Can you work these out from the drawing? Everything is in mm from the part's minimum corner. Give positions to 0.01 mm unless a question says otherwise; leave off trailing zeros. Loops run counter-clockwise (first coordinate to the right, second up) from the corner with the lowest first, then second, coordinate; pieces in that order, holes last.
Q1. If we section it at C-C (z = 94): Please give me the cut outline in (x, y).
Q2. I need wall thicknesses on line 1 (Y direction, x = 18, z = 3); line 2 (X direction, y = 17.5, z = 67); line 3 (X direction, y = 21, z = 73). Which ranges of each line are inside material? Lowest first, please.
Q3. If we section it at A-A (y = 18): Please give me the cut outline in (x, z).
Q4. If we section it at D-D (y = 32): Please give me the cut outline in (x, z).
Q5. If we section it at B-B (x = 20.5): Please give me the cut outline in (y, z), plus the area to 3 significant figures.
Q6. Will these pins go through, and if not, where does the flat tip stop? P1, Ø10, axis at x = 25.5, z = 93.5, coming from the +Y side; P2, Ø8, axis at x = 15.5, y = 25, coming from the -Z side; P3, Ø6, axis at y = 27.5, z = 32, coming from the -X side; P4, Ø1.5, axis at x = 32, y = 17.5, coming from the -Z side.
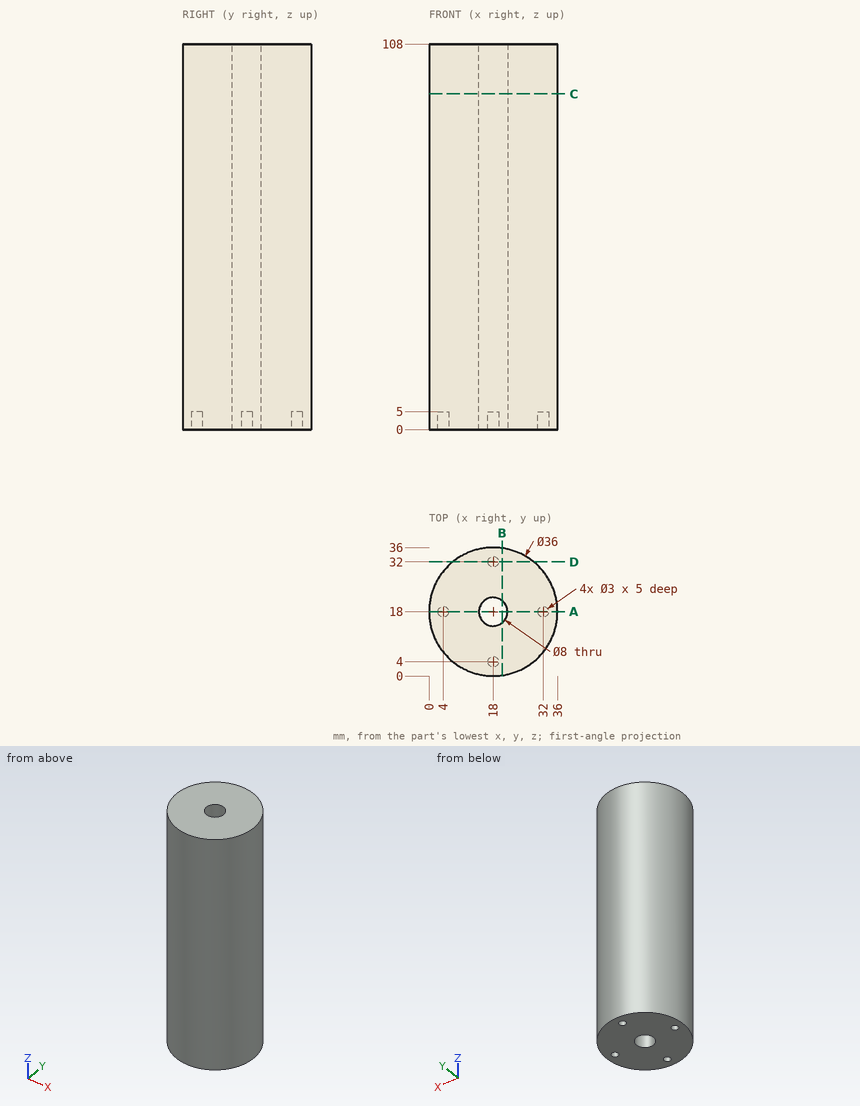
Check sheet entries:
1. outline: circle Ø36 at (18, 18); hole circle Ø8 at (18, 18)
2. line 1: y = 0 to 2.5, 5.5 to 14, 22 to 30.5, 33.5 to 36
2. line 2: x = 0.01 to 14.03, 21.97 to 35.99
2. line 3: x = 0.25 to 15.35, 20.65 to 35.75
3. outline: (0, 0) - (2.5, 0) - (2.5, 5) - (5.5, 5) - (5.5, 0) - (14, 0) - (14, 108) - (0, 108) - close; (22, 0) - (30.5, 0) - (30.5, 5) - (33.5, 5) - (33.5, 0) - (36, 0) - (36, 108) - (22, 108) - close
4. outline: (6.69, 0) - (16.5, 0) - (16.5, 5) - (19.5, 5) - (19.5, 0) - (29.31, 0) - (29.31, 108) - (6.69, 108) - close
5. outline: (0.17, 0) - (14.88, 0) - (14.88, 108) - (0.17, 108) - close; (21.12, 0) - (35.83, 0) - (35.83, 108) - (21.12, 108) - close
5. area: 3,180 mm2
6. P1: stops at y = 35.83
6. P2: stops at z = 0
6. P3: stops at x = 1.21
6. P4: stops at z = 5
